Autodesk Inventor part; units mm, degrees
ref_plane "YZ Plane" through (0, 0, 0) normal (1, 0, 0) x (0, 1, 0)
ref_plane "XZ Plane" through (0, 0, 0) normal (0, 1, 0) x (-1, 0, 0)
ref_plane "XY Plane" through (0, 0, 0) normal (0, 0, 1) x (1, 0, 0)
sketch "Sketch1" plane through (0, 0, 0) normal (0, 1, 0) x (-1, 0, 0)
  line L0 (0, 0) -> (10, 0)
  line L1 (10, 0) -> (10, -27)
  line L2 (10, -27) -> (0, -27)
  line L3 (0, -27) -> (0, 0)
  dimension "d0" = 10
  dimension "d1" = 27
extrude "Extrusion1" add sketch "Sketch1" along normal blind 10
sketch "Sketch2" plane through (0, 10, 0) normal (0, 1, 0) x (1, 0, 0)
  line L0 (-10, 27) -> (-10, 0)
  line L1 (-10, 0) -> (-10, 5)
  circle A0 centre (-5, 5) radius 2.55
  point P0 (0, 0)
  dimension "d4" = 5
  dimension "d5" = 5.1
extrude "Extrusion2" cut sketch "Sketch2" against normal blind 10
sketch "Sketch4" plane through (0, 10, 0) normal (0, 1, 0) x (1, 0, 0)
  line L0 (0, 27) -> (-10, 27)
  line L1 (-10, 27) -> (-10, 0)
  line L2 (0, 27) -> (-10, 27)
  line L3 (-10, 27) -> (-10, 0)
  line L4 (-10, 0) -> (0, 0)
  line L5 (0, 0) -> (0, 27)
  point P0 (0, 0)
  dimension "d13" = 27
extrude "Extrusion4" cut sketch "Sketch4" against normal blind 7
properties part number "Raket_Arme_Motor"
CAD build for the part. Positions are in the model's coordinates, mm. Coordinates: 2 decimals unless noted, no trailing zeros. Order: outer loops, then holes, each group sorted by start corner. A loop starts at its lowest first (then second) coordinate and runs counter-clockwise, first axis right, second up. Notation, with made-up numbers: (49.25, -12.75) -> (60.25, -12.75) arc R31 ccw to (60.25, 19.25) -> close; hole circle Ø2 at (70.5, -33). An arc over 180 degrees is marked (long way). Use one line per item in the form item = value. Start each with the question number.
1) Pull direction Z, two halves, no side cores. Call faces 1 (the flat face through (-5, 1, -27)), 2 (the flat face through (-5, 0, -13)), 3 (the cylindrical face through (-2.57, 1.52, -5.77)): +Z half, -Z half, draft (parallel to the pull), parting line (faces both ways), or undercut.
2) Band-saw the part on B-B on x = -5.5. Give the cut face in (y, z), then the cut area to 3 significant figures.
3) Band-saw the part on C-C on y = 0.3. Give the cut face in (x, z).
4) Band-saw the part on A-A on z = -5. Give the cut face in (x, y), then the cut area to 3 significant figures.
5) Drill centre lines: L1, parallel to X at y = 1.05, z = -5; L2, parallel to Z at x = -5, y = 1.75; L3, parallel to X at y = 1.25, z = -3.5. Where is each one in solid material? Low to high. Write a range as [from, to].
Entries:
q1.face_1 = -Z half
q1.face_2 = draft
q1.face_3 = undercut
q2.outline = (0, -27) -> (3, -27) -> (3, -7.5) -> (0, -7.5) -> close; (0, -2.5) -> (3, -2.5) -> (3, 0) -> (0, 0) -> close
q2.area = 66.0 mm2
q3.outline = (-10, -27) -> (0, -27) -> (0, 0) -> (-10, 0) -> close; hole circle Ø5.1 at (-5, -5)
q4.outline = (-10, 0) -> (-7.55, 0) -> (-7.55, 3) -> (-10, 3) -> close; (-2.45, 0) -> (0, 0) -> (0, 3) -> (-2.45, 3) -> close
q4.area = 14.7 mm2
q5.L1 = [-10, -7.55], [-2.45, 0]
q5.L2 = [-27, -7.55], [-2.45, 0]
q5.L3 = [-10, -7.06], [-2.94, 0]
